Here's how the part is built. I have some questions about the finished solid (model axes, mm). Face numbers are marked on the shaded views. A direction names the side the tool comes from. Coordinates: 2 decimals unless noted, no trailing zeros. Order: outer loops, then holes, each group sorted by start corner. A loop starts at its lowest first (then second) coordinate and runs counter-clockwise, first axis right, second up. Notation, with made-up numbers: (51, 29.5) - (79, 29.5) arc R15 cw to (79, 48.5) - close; hole circle Ø2 at (-33.75, 9). An arc over 180 degrees is marked (long way). Answer in a Markdown table with one row per item. Add a question column.
Item 1: Will these pins go through, and if not, where does the flat tip stop? pin 1 Ø3 at (x, z) = (0, 0) entering from -Y; pin 2 Ø1.3 at (x, z) = (0, 0) entering from +Y; pin 3 Ø1.5 at (x, z) = (-2, 4) entering from +Y.
Item 2: I want a section at C-C (y = 2.75). Please give me the cut outline in (x, z).
Item 3: On a 3-axis mill with a long thin cutter (end or side, diameter ignored), from which of +Z, -Z, +X, -X, +Y, -Y can I reach the whole of each face in a straight line? I mean the marked faces 1 and 2. Say none if no direction works.
Item 4: I want a section at B-B (x = 0). Please give me the cut outline in (y, z), plus the area to 3 significant figures.
Item 5: Thinking about a two-plate mould opening in Z: for the marked faces 3, 4 and 5, which applies, +Z half, -Z half, draft (parallel to the pull), parting line (faces both ways), or undercut?
Item 6: I want a section at D-D (x = -2.25). Please give me the cut outline in (y, z).
Item 7: I want a section at A-A (z = 0). Please give me the cut outline in (x, y).
Item 8: If I drill on line 1 along X through (y, z) = (2.15, 0); line 2 along X through (y, z) = (0.55, 0); line 3 along Y through (x, z) = (-1, -4), over which ranges is the centre line in solid material (lowest first)? Write a range as from..to.
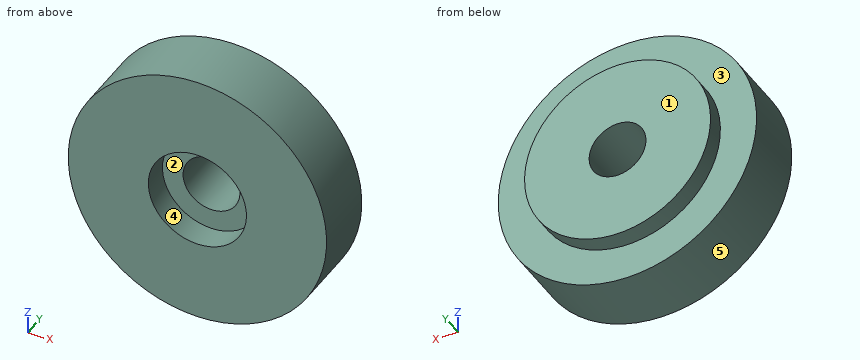
```python
from build123d import *

# Parameters (mm, degrees)
SKETCH_1_R          = 5
EXTRUDE_1_DEPTH     = 2.5
SKETCH_2_R          = 3.6
EXTRUDE_2_DEPTH     = 0.7
SKETCH_3_R          = 1.1
CUT_EXTRUDE_1_DEPTH = 8.761443165
SKETCH_4_R          = 1.9
CUT_EXTRUDE_2_DEPTH = 1


with BuildPart() as part:
    # 草图1 → 凸台-拉伸1 (new body)
    with BuildSketch(Plane(origin=(0, 0, 0), x_dir=(1, 0, 0), z_dir=(0, 1, 0))):
        with Locations(Location((0, 0, 0), (0, 0, 270))):
            Circle(SKETCH_1_R)
    extrude(amount=EXTRUDE_1_DEPTH)

    # 草图2 → 凸台-拉伸2 (add)
    with BuildSketch(Plane(origin=(0, 2.5, 0), x_dir=(1, 0, 0), z_dir=(0, 1, 0))):
        with Locations(Location((0, 0, 0), (0, 0, 270))):
            Circle(SKETCH_2_R)
    extrude(amount=EXTRUDE_2_DEPTH)

    # 草图3 → 切除-拉伸1 (cut, through all)
    with BuildSketch(Plane(origin=(0, 3.2, 0), x_dir=(1, 0, 0), z_dir=(0, 1, 0))):
        with Locations(Location((0, 0, 0), (0, 0, 270))):
            Circle(SKETCH_3_R)
    extrude(amount=-CUT_EXTRUDE_1_DEPTH, mode=Mode.SUBTRACT)

    # 草图4 → 切除-拉伸2 (cut)
    with BuildSketch(Plane.XZ):
        with Locations(Location((0, 0, 0), (0, 0, 270))):
            Circle(SKETCH_4_R)
    extrude(amount=-CUT_EXTRUDE_2_DEPTH, mode=Mode.SUBTRACT)


solid = part.part
```
Values follow:
| question | item | result |
|---|---|---|
| 1 | pin 1 | stops at y = 1 |
| 1 | pin 2 | passes through |
| 1 | pin 3 | stops at y = 2.5 |
| 2 | outline | circle Ø7.2 at (0, 0); hole circle Ø2.2 at (0, 0) |
| 3 | face 1 | +Z, -Z, +X, -X, +Y |
| 3 | face 2 | -Y |
| 4 | outline | (0, -5) - (2.5, -5) - (2.5, -3.6) - (3.2, -3.6) - (3.2, -1.1) - (1, -1.1) - (1, -1.9) - (0, -1.9) - close; (0, 1.9) - (1, 1.9) - (1, 1.1) - (3.2, 1.1) - (3.2, 3.6) - (2.5, 3.6) - (2.5, 5) - (0, 5) - close |
| 4 | area | 21.4 mm^2 |
| 5 | face 3 | draft |
| 5 | face 4 | undercut |
| 5 | face 5 | parting line |
| 6 | outline | (0, -4.47) - (2.5, -4.47) - (2.5, -2.81) - (3.2, -2.81) - (3.2, 2.81) - (2.5, 2.81) - (2.5, 4.47) - (0, 4.47) - close |
| 7 | outline | (-5, 0) - (-1.9, 0) - (-1.9, 1) - (-1.1, 1) - (-1.1, 3.2) - (-3.6, 3.2) - (-3.6, 2.5) - (-5, 2.5) - close; (1.1, 1) - (1.9, 1) - (1.9, 0) - (5, 0) - (5, 2.5) - (3.6, 2.5) - (3.6, 3.2) - (1.1, 3.2) - close |
| 8 | line 1 | x = -5..-1.1, 1.1..5 |
| 8 | line 2 | x = -5..-1.9, 1.9..5 |
| 8 | line 3 | y = 0..2.5 |
